Model file for the job. Use its own axes, mm. Face numbers are marked on the shaded views. Give positions to 0.01 mm unless a question says otherwise; leave off trailing zeros. Write each loop counter-clockwise with the first axis right and the second up, starting at its lowest first coordinate (ties: lowest second). Pieces come first, ordered by that corner, then holes. Notation, with made-up numbers: (53, 30.25) - (110, 30.25) arc R18 cw to (110, 48.25) - close; hole circle Ø8 at (27, -29.5). An arc over 180 degrees is marked (long way). One line per item, written item: value. Start each with the question number.
(1) Drop a flat-ended pin along its axis: P1, Ø2, axis at x = 48.5, y = -8, coming from the +Z side. Give the stop position or say it passes through.
(2) Probe L1, parallel to X at y = -6.35, z = 116.1; L2, parallel to Y at x = 50, z = 118; L3, parallel to X at y = -6.35, z = 118.4. List the from-to ranges inside material, lowest first.
(3) Mould opens along X. For the marked faces 1, 2 and 3 say: pulls with the +X half, pulls with the -X half, needs draft (parallel to the pull), parting line crosses it, or undercut.
(4) Cut at B-B, the plane y = -11. List the corners of the cut face in (x, z) (3 decimals).
(5) Cut at A-A, the plane x = 0. List the corners of the cut face in (y, z), and give its area (3 significant figures).
(6) Cut at D-D, the plane x = 25. List the corners of the cut face in (y, z).
(7) Cut at C-C, the plane z = 112. List the corners of the cut face in (x, y), and give its area (3 significant figures).
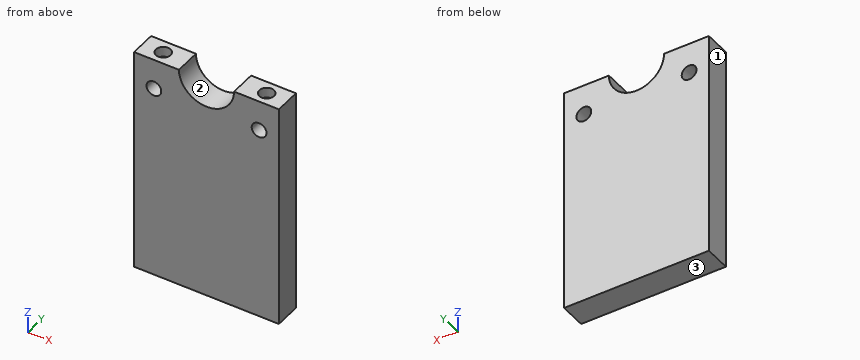
from build123d import *

# Parameters (mm, degrees)
SKETCH026_R  = 3.571875
PAD026_DEPTH = 6
SKETCH025_R  = 3.571875
PAD025_DEPTH = 6
SKETCH024_R  = 3.571875
PAD024_DEPTH = 50
SKETCH023_R  = 3.571875
PAD023_DEPTH = 33.7
PAD001_DEPTH = 12.7


with BuildPart() as body026:
    # Sketch026 → Pad026 (new body)
    with BuildSketch(Plane.XY):
        Circle(SKETCH026_R)
    extrude(amount=PAD026_DEPTH)


with BuildPart() as body026_1:
    # Body026 placement: moved
    add(body026.part.moved(Location((150, -6.35, 115))))


with BuildPart() as body025:
    # Sketch025 → Pad025 (new body)
    with BuildSketch(Plane.XY):
        Circle(SKETCH025_R)
    extrude(amount=PAD025_DEPTH)


with BuildPart() as body025_1:
    # Body025 placement: moved
    add(body025.part.moved(Location((100, -6.35, 115))))


with BuildPart() as body024:
    # Sketch024 → Pad024 (new body)
    with BuildSketch(Plane.XZ):
        Circle(SKETCH024_R)
    extrude(amount=PAD024_DEPTH)


with BuildPart() as body024_1:
    # Body024 placement: moved
    add(body024.part.moved(Location((50.4341, 10, 105.316))))


with BuildPart() as body023:
    # Sketch023 → Pad023 (new body)
    with BuildSketch(Plane.XZ):
        Circle(SKETCH023_R)
    extrude(amount=PAD023_DEPTH)


with BuildPart() as body023_1:
    # Body023 placement: moved
    add(body023.part.moved(Location((-0.434083, 5, 105.316))))


with BuildPart() as bracelower001:
    # Sketch001 → Pad001 (new body)
    with BuildSketch(Plane.XZ):
        with BuildLine():
            Line((0, 0), (0, 110))
            Line((0, 110), (21.675, 110))
            ThreePointArc((21.675, 110), (35, 96.674972), (48.325, 110))
            Line((48.325, 110), (70, 110))
            Line((70, 110), (70, 0))
            Line((70, 0), (0, 0))
        make_face()
    extrude(amount=PAD001_DEPTH)


with BuildPart() as bracelower001_1:
    # Body001 placement: moved
    add(bracelower001.part.moved(Location((-10, 0, 10))))

    # Cut016: cut Body023
    add(body023_1.part, mode=Mode.SUBTRACT)

    # Cut017: cut Body024
    add(body024_1.part, mode=Mode.SUBTRACT)


with BuildPart() as bracelower001_2:
    # Cut017 placement: moved
    add(bracelower001_1.part.moved(Location((100, 0, 0))))

    # Cut018: cut Body025
    add(body025_1.part, mode=Mode.SUBTRACT)

    # Cut019: cut Body026
    add(body026_1.part, mode=Mode.SUBTRACT)


with BuildPart() as bracelower001_3:
    # Cut019 placement: moved
    add(bracelower001_2.part.moved(Location((-100, 0, 0))))


solid = bracelower001_3.part
Answers follow:
1. P1: stops at z = 115
2. L1: x = -10 to -3.57, 3.57 to 12.26, 37.74 to 46.43, 53.57 to 60
2. L2: y = -12.7 to -9.92, -2.78 to 0
2. L3: x = -10 to -3.57, 3.57 to 11.77, 38.23 to 46.43, 53.57 to 60
3. face 1: pulls with the -X half
3. face 2: undercut
3. face 3: needs draft
4. outline: (-10, 10) - (60, 10) - (60, 120) - (38.325, 120) arc R13.325 cw to (11.675, 120) - (-10, 120) - close; hole circle Ø7.144 at (-0.434, 105.316); hole circle Ø7.144 at (50.434, 105.316)
5. outline: (-12.7, 10) - (0, 10) - (0, 101.77) - (-12.7, 101.77) - close; (-12.7, 108.86) - (0, 108.86) - (0, 120) - (-2.78, 120) - (-2.78, 115) - (-9.92, 115) - (-9.92, 120) - (-12.7, 120) - close
5. area: 1,270 mm²
6. outline: (-12.7, 10) - (0, 10) - (0, 106.67) - (-12.7, 106.67) - close
7. outline: (-10, -12.7) - (14.34, -12.7) - (14.34, 0) - (-10, 0) - close; (35.66, -12.7) - (60, -12.7) - (60, 0) - (35.66, 0) - close
7. area: 618 mm²
